Here's how the part is built. I have some questions about the finished solid (model axes, mm). A direction names the side the tool comes from. Round coordinates to 2 decimals unless told otherwise and drop trailing zeros. Write each loop counter-clockwise with the first axis right and the second up, starting at its lowest first coordinate (ties: lowest second). Pieces come first, ordered by that corner, then holes. Notation, with made-up numbers: M -13.5,89 L 1.5,89 A17 cw 1.5,118 Z; hole C 48.25,48 d3. An arc over 180 degrees is marked long. Write item = value, one per line. Start each with the question number.
(1) I need wall thicknesses on line 1 along X through (y, z) = (7, 15); line 2 along X through (y, z) = (11, 20.5); line 3 along Z through (x, y) = (1.5, 4). Which ranges of each line are inside material? Lowest first, please.
(2) On a 3-axis mill with a long thin cutter (end or side, diameter ignored), from which of +Z, -Z, +X, -X, +Y, -Y can I reach the whole of each face in a straight line? I mean faces 1 (the flat face through (-12.82, 21.15, 36.41)), 2 (the flat face through (0, 16, 22)), 3 (the flat face through (-29, 16, 9)), 4 (the flat face through (-6.5, 16, 10)). Say none if no direction works.
(3) If we mould it in two halves opening along X, with no side actions, what happens to faces 5 (the flat face through (-26, 16, 22)), 6 (the flat face through (3, 16, 9)), 7 (the flat face through (-13, 16, 20))? For each: released by +X, released by -X, zero draft, split by the parting line, or undercut.
(4) I want a section at C-C (x = -4). List the corners of the cut face in (y, z) for me.
(5) I want a section at D-D (y = 27). List the corners of the cut face in (x, z) for me.
(6) I want a section at B-B (y = 3). List the corners of the cut face in (x, z) for me, and give its area (3 significant figures).
(7) Will these pins go through, and if not, where does the flat tip stop? pin 1 Ø16 at (y, z) = (23, 22) entering from +X; pin 2 Ø2 at (x, y) = (-29.5, 10) entering from +Z; pin 3 Ø4 at (y, z) = (16, 26.5) entering from -X.
(8) I want a section at A-A (z = 6). List the corners of the cut face in (x, y) for me, and give its area (3 significant figures).
```python
from build123d import *

# Parameters (mm, degrees)
BOSS_EXTRUDE2_DEPTH = 26
SKETCH2_W           = 9
SKETCH2_H           = 32
BOSS_EXTRUDE3_DEPTH = 7
SKETCH3_W           = 9
SKETCH3_H           = 32
BOSS_EXTRUDE4_DEPTH = 7
SKETCH4_W           = 13
SKETCH4_H           = 20
CUT_EXTRUDE2_DEPTH  = 34


with BuildPart() as part:
    # Sketch1 → Boss-Extrude2 (new body)
    with BuildSketch(Plane(origin=(0, 0, 0), x_dir=(0, 0, -1), z_dir=(1, 0, 0))):
        Polygon((-43, 0), (0, 0), (0, 32), (-30, 32), (-43, 10), align=None)
    extrude(amount=-BOSS_EXTRUDE2_DEPTH)

    # Sketch2 → Boss-Extrude3 (add)
    with BuildSketch(Plane(origin=(0, 0, 0), x_dir=(0, 0, -1), z_dir=(1, 0, 0))):
        with Locations((-4.5, 16)):
            Rectangle(SKETCH2_W, SKETCH2_H)
    extrude(amount=BOSS_EXTRUDE3_DEPTH)

    # Sketch3 → Boss-Extrude4 (add)
    with BuildSketch(Plane.ZY.offset(26)):
        with Locations((4.5, 16)):
            Rectangle(SKETCH3_W, SKETCH3_H)
    extrude(amount=BOSS_EXTRUDE4_DEPTH)

    # Sketch4 → Cut-Extrude2 (cut)
    with BuildSketch(Plane(origin=(0, 32, 0), x_dir=(1, 0, 0), z_dir=(0, 1, 0))):
        with Locations((-13, -10)):
            Rectangle(SKETCH4_W, SKETCH4_H)
    extrude(amount=-CUT_EXTRUDE2_DEPTH, mode=Mode.SUBTRACT)


solid = part.part
```
Returned:
q1.line_1 = -26 to -19.5, -6.5 to 0
q1.line_2 = -26 to 0
q1.line_3 = 0 to 9
q2.face_1 = +Z, +X, -X, +Y
q2.face_2 = +Z, +X, +Y, -Y
q2.face_3 = +Z, -X, +Y, -Y
q2.face_4 = -Z, +Y, -Y
q3.face_5 = released by -X
q3.face_6 = zero draft
q3.face_7 = undercut
q4.outline = M 0,0 L 32,0 L 32,30 L 10,43 L 0,43 Z
q5.outline = M -33,0 L -19.5,0 L -19.5,20 L -6.5,20 L -6.5,0 L 7,0 L 7,9 L 0,9 L 0,32.95 L -26,32.95 L -26,9 L -33,9 Z
q6.outline = M -33,0 L -19.5,0 L -19.5,20 L -6.5,20 L -6.5,0 L 7,0 L 7,9 L 0,9 L 0,43 L -26,43 L -26,9 L -33,9 Z
q6.area = 984 mm²
q7.pin_1 = 0
q7.pin_2 = 9
q7.pin_3 = -26
q8.outline = M -33,0 L -19.5,0 L -19.5,32 L -33,32 Z; M -6.5,0 L 7,0 L 7,32 L -6.5,32 Z
q8.area = 864 mm²
